Here's how the part is built. I have some questions about the finished solid (model axes, mm). A direction names the side the tool comes from. Coordinates: 2 decimals unless noted, no trailing zeros. Write each loop counter-clockwise with the first axis right and the second up, starting at its lowest first coordinate (ties: lowest second). Pieces come first, ordered by that corner, then holes. Notation, with made-up numbers: M 1,37.25 L 20,37.25 A31 ccw 20,72.25 Z; hole C 17,20.25 d1. An arc over 180 degrees is marked long. Use a Markdown table: item, result.
```python
from build123d import *

# Parameters (mm, degrees)
F0_R     = 8.5
F1_DEPTH = 40
F2_T     = -2
F3_SIZE  = 1.99999
F5_DEPTH = 1.5


# Not quite as in the source:
# - a fillet or chamfer is up to 0.001 mm smaller than in the source, because OpenCascade refuses the exact size


with BuildPart() as f1:
    # F0 (on Top) → F1 (new body)
    with BuildSketch(Plane.XY):
        Circle(F0_R)
    extrude(amount=F1_DEPTH)

    # F2
    f2_openings = [f1.faces().sort_by_distance(p)[0] for p in [
        (0, 0, 40),
    ]]
    offset(amount=F2_T, openings=f2_openings)

    # F3 (size 2 in the source; OpenCascade refuses exactly that, so slightly less here)
    f3_edges = [f1.edges().sort_by_distance(p)[0] for p in [
        (-6.5, 0, 40),
    ]]
    chamfer(f3_edges, length=F3_SIZE)

    # F4 (on Front) → F5 (join, symmetric)
    with BuildSketch(Plane.XZ):
        Polygon((-8.2697293678, 1.3648961653), (-8.2697293678, 7.3648961653), (-10.9697293678, 7.3648961653), (-10.9697293678, 1.3648961653), (-10.2286748588, 1.3648961653), (-10.2286748588, 4.6420348808), (-9.2178666964, 4.6420348808), (-9.2178666964, 1.3648961653), align=None)
        Polygon((10.9697293678, 7.3648961653), (8.2697293678, 7.3648961653), (8.2697293678, 1.3648961653), (9.2178666964, 1.3648961653), (9.2178666964, 4.6420348808), (10.2286748588, 4.6420348808), (10.2286748588, 1.3648961653), (10.9697293678, 1.3648961653), align=None)
    extrude(amount=F5_DEPTH, both=True)


solid = f1.part
```
1. Suppose I cut it at C-C on z = 30.5. Write out the boundary of the cut face in (x, y), and give its area (3 significant figures).
Answers follow:
| item | result |
|---|---|
| outline | C 0,0 d17; hole C 0,0 d13 |
| area | 94.2 mm2 |
2. Will these pins go through, and if not, where does the flat tip stop? pin 1 Ø0.8 at (x, y) = (9, 0) entering from +Z; pin 2 Ø6 at (y, z) = (2.5, 21.5) entering from -X; pin 3 Ø3 at (x, z) = (9, 3) entering from +Y.
Answers follow:
| item | result |
|---|---|
| pin 1 | stops at z = 7.36 |
| pin 2 | stops at x = -8.5 |
| pin 3 | stops at y = 4 |
3. We'd pull the mould along X, two halves only. Please class faces 5 (the face through (-10, -1.5, 5)), 6 (the face through (0, 0, 2)), 7 (the face through (8.11, 2.55, 19.72)): +X half, -X half, draft (parallel to the pull), parting line (faces both ways), or undercut.
Answers follow:
| item | result |
|---|---|
| face 5 | draft |
| face 6 | undercut |
| face 7 | parting line |
4. I need wall thicknesses on probe 1 along Y at (x, z) = (0, 12.5); probe 2 along X at (y, z) = (2.5, 7.5). Which ranges of each line are inside material? Lowest first, please.
Answers follow:
| item | result |
|---|---|
| probe 1 | y = -8.5 to -6.5, 6.5 to 8.5 |
| probe 2 | x = -8.12 to -6, 6 to 8.12 |
5. Which directions (+Z, -Z, +X, -X, +Y, -Y) give clear straight access to the entire face, cutting with the end or side of a thin tool? Please do faces 1 (the face through (-5.158, -3.955, 19.748)), 2 (the face through (10, -1.5, 5)), 3 (the face through (9.218, 0, 3)), 4 (the face through (-10, 1.5, 5)).
Answers follow:
| item | result |
|---|---|
| face 1 | +Z |
| face 2 | +Z, -Z, +X, -Y |
| face 3 | -Z, +Y, -Y |
| face 4 | +Z, -Z, -X, +Y |
